from build123d import *

# Parameters (mm, degrees)
BOSS_EXTRUDE4_DEPTH = 8.5
BOSS_EXTRUDE5_DEPTH = 8.8
CUT_EXTRUDE1_DEPTH  = 1.5
CUT_EXTRUDE2_REACH  = 35.269
SKETCH7_R           = 1.1303


with BuildPart() as part:
    # Sketch4 → Boss-Extrude4 (new body)
    with BuildSketch(Plane.XY):
        Polygon((0, 0), (0, 3), (5.8, 3), (5.8, 11.5), (20.8, 11.5), (20.8, 3), (26.6, 3), (26.6, 0), (19.3, 0), (19.3, 10), (7.3, 10), (7.3, 0), align=None)
    extrude(amount=BOSS_EXTRUDE4_DEPTH)

    # Sketch5 → Boss-Extrude5 (add)
    with BuildSketch(Plane.XY.offset(8.5)):
        Polygon((7.3, 0), (7.3, 10), (19.3, 10), (19.3, 0), (20.8, 0), (20.8, 11.5), (5.8, 11.5), (5.8, 0), align=None)
    extrude(amount=BOSS_EXTRUDE5_DEPTH)

    # Sketch6 → Cut-Extrude1 (cut)
    with BuildSketch(Plane(origin=(0, 3, 0), x_dir=(1, 0, 0), z_dir=(0, 1, 0))):
        Polygon((24.898076211, -5.75), (22.3, -7.25), (19.701923789, -5.75), (19.701923789, -2.75), (22.3, -1.25), (24.898076211, -2.75), align=None)
        Polygon((4.3, -7.25), (6.898076211, -5.75), (6.898076211, -2.75), (4.3, -1.25), (1.701923789, -2.75), (1.701923789, -5.75), align=None)
    extrude(amount=-CUT_EXTRUDE1_DEPTH, mode=Mode.SUBTRACT)

    # Sketch7 → Cut-Extrude2 (cut, up to next)
    with BuildSketch(Plane(origin=(0, 1.5, 0), x_dir=(1, 0, 0), z_dir=(0, 1, 0)), mode=Mode.PRIVATE) as cut_extrude2_sk1:
        with Locations(Location((4.3, -4.25, 0), (0, 0, 270))):
            Circle(SKETCH7_R)
    cut_extrude2_tool1 = extrude(cut_extrude2_sk1.sketch, amount=-CUT_EXTRUDE2_REACH, mode=Mode.PRIVATE) & part.part
    # Sketch7 → Cut-Extrude2 (cut, up to next)
    with BuildSketch(Plane(origin=(0, 1.5, 0), x_dir=(1, 0, 0), z_dir=(0, 1, 0)), mode=Mode.PRIVATE) as cut_extrude2_sk2:
        with Locations(Location((22.3, -4.25, 0), (0, 0, 270))):
            Circle(SKETCH7_R)
    cut_extrude2_tool2 = extrude(cut_extrude2_sk2.sketch, amount=-CUT_EXTRUDE2_REACH, mode=Mode.PRIVATE) & part.part
    add(cut_extrude2_tool1.solids().sort_by_distance((4.3, 1.5, 4.25))[0], mode=Mode.SUBTRACT)
    add(cut_extrude2_tool2.solids().sort_by_distance((22.3, 1.5, 4.25))[0], mode=Mode.SUBTRACT)


solid = part.part
Could you check a few things on this model? Use its own coordinates, in mm. A direction names the side the tool comes from. Round coordinates to 2 decimals unless told otherwise and drop trailing zeros. Write each loop counter-clockwise with the first axis right and the second up, starting at its lowest first coordinate (ties: lowest second). Pieces come first, ordered by that corner, then holes. Notation, with made-up numbers: (54.25, -27.75) - (111.25, -27.75) arc R14 cw to (111.25, -16.75) - close; hole circle Ø4 at (33, -13). An arc over 180 degrees is marked (long way). Put each result on its own line as item: value. Start each with the question number.
(1) I want a section at B-B, the plane z = 4.25. Please give me the cut outline in (x, y), plus the area to 3 significant figures.
(2) Thinking about a two-plate mould opening in X: for faces 1 (the flat face through (3, 2, 2)), 2 (the flat face through (5.6, 2.3, 2)), 3 (the flat face through (0, 1, 4)), 4 (the flat face through (13, 11.5, 9)), which applies, released by +X, released by -X, zero draft, split by the parting line, or undercut?
(3) I want a section at A-A, the plane y = 0.5. Please give me the cut outline in (x, z), plus the area to 3 significant figures.
(4) For faces 5 (the flat face through (1, 3, 4)), 6 (the flat face through (24.898, 2, 4)), 7 (the flat face through (3, 1.5, 4)), 8 (the flat face through (19.3, 5, 9)), which set-ups out of +Z, -Z, +X, -X, +Y, -Y let a thin tool reach every point of the face, with its end or its side?
(5) Will these pins go through, and if not, where does the flat tip stop? pin 1 (3 mm diameter, centred on x = 22.5, z = 4.5, fed in from +Y); pin 2 (1.5 mm diameter, centred on y = 4, z = 10.5, fed in from -X); pin 3 (1.5 mm diameter, centred on x = 1.5, y = 2, fed in from +Z).
(6) I need wall thicknesses on probe 1 along X at (y, z) = (1.05, 4.25); probe 2 along X at (y, z) = (6.75, 1); probe 3 along Y at (x, z) = (10, 5). Which ranges of each line are inside material? Lowest first, please.
(7) I want a section at C-C, the plane y = 5.25. Please give me the cut outline in (x, z).
(8) I want a section at D-D, the plane z = 15.25. Please give me the cut outline in (x, y), plus the area to 3 significant figures.
Here are the results:
1. outline: (0, 0) - (3.17, 0) - (3.17, 1.5) - (1.7, 1.5) - (1.7, 3) - (0, 3) - close; (5.43, 0) - (7.3, 0) - (7.3, 10) - (19.3, 10) - (19.3, 0) - (21.17, 0) - (21.17, 1.5) - (19.7, 1.5) - (19.7, 3) - (20.8, 3) - (20.8, 11.5) - (5.8, 11.5) - (5.8, 3) - (6.9, 3) - (6.9, 1.5) - (5.43, 1.5) - close; (23.43, 0) - (26.6, 0) - (26.6, 3) - (24.9, 3) - (24.9, 1.5) - (23.43, 1.5) - close
1. area: 64.9 mm^2
2. face 1: undercut
2. face 2: undercut
2. face 3: released by -X
2. face 4: zero draft
3. outline: (0, 0) - (7.3, 0) - (7.3, 17.3) - (5.8, 17.3) - (5.8, 8.5) - (0, 8.5) - close; (19.3, 0) - (26.6, 0) - (26.6, 8.5) - (20.8, 8.5) - (20.8, 17.3) - (19.3, 17.3) - close; hole circle Ø2.26 at (4.3, 4.25); hole circle Ø2.26 at (22.3, 4.25)
3. area: 142 mm^2
4. face 5: +Z, -Z, -X, +Y
4. face 6: +Y
4. face 7: none
4. face 8: +Z, -Z, -Y
5. pin 1: stops at y = 1.5
5. pin 2: stops at x = 5.8
5. pin 3: stops at z = 8.5
6. probe 1: x = 0 to 3.17, 5.43 to 7.3, 19.3 to 21.17, 23.43 to 26.6
6. probe 2: x = 5.8 to 7.3, 19.3 to 20.8
6. probe 3: y = 10 to 11.5
7. outline: (5.8, 0) - (7.3, 0) - (7.3, 17.3) - (5.8, 17.3) - close; (19.3, 0) - (20.8, 0) - (20.8, 17.3) - (19.3, 17.3) - close
8. outline: (5.8, 0) - (7.3, 0) - (7.3, 10) - (19.3, 10) - (19.3, 0) - (20.8, 0) - (20.8, 11.5) - (5.8, 11.5) - close
8. area: 52.5 mm^2
